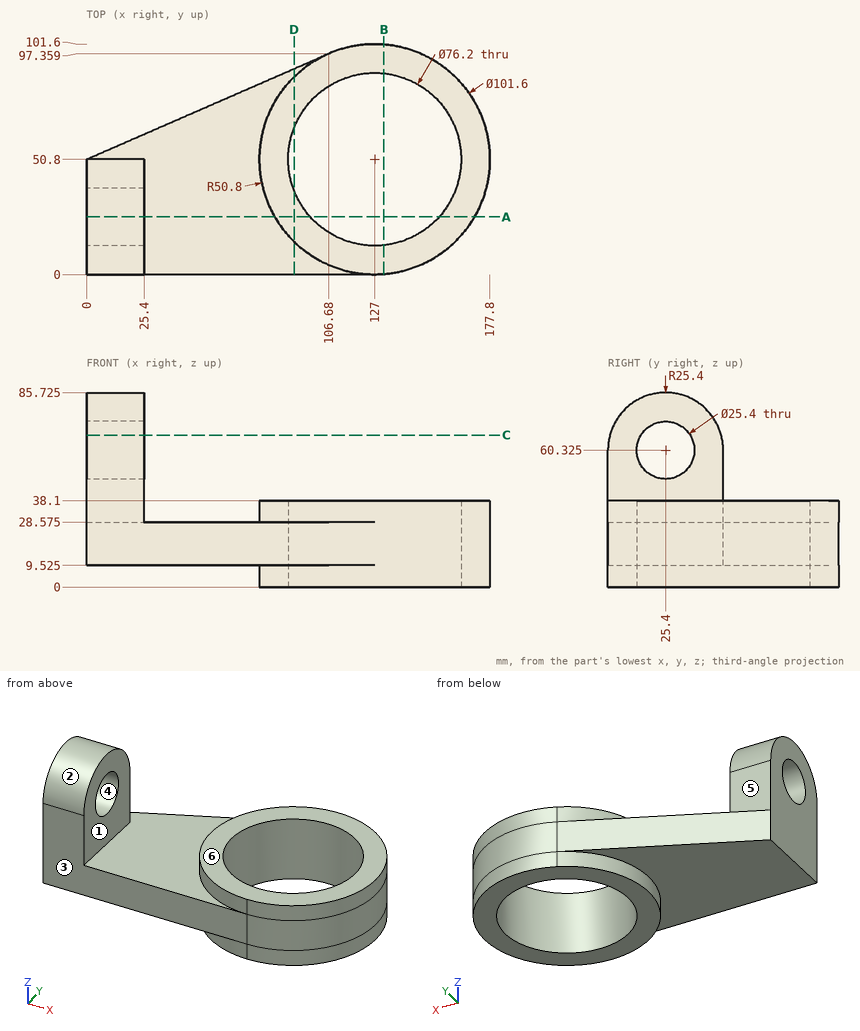
Design review of the part shown in the three views and the two pictorial views. Dimensions are in mm from the part's minimum x, y and z. A direction names the side the tool comes from. Coordinates: 2 decimals unless noted, no trailing zeros. Order: outer loops, then holes, each group sorted by start corner. A loop starts at its lowest first (then second) coordinate and runs counter-clockwise, first axis right, second up. Notation, with made-up numbers: (-2.5, 85.5) -> (39.5, 85.5) arc R21 ccw to (39.5, 106.5) -> close; hole circle Ø7 at (41, 42). An arc over 180 degrees is marked (long way). Use one line per item in the form item = value. Start each with the question number.
(1) The part is to be moulded in two halves that separate along Y. For the marked faces 3, 4, 5 and 6, say which applies: +Y half, -Y half, draft (parallel to the pull), parting line (faces both ways), or undercut.
(2) Insertion check: pin 1 (6 mm diameter, centred on x = 56, y = 54, fed in from -Z) (3 decimals); pin 2 (6 mm diameter, centred on y = 31, z = 10, fed in from +X); pin 3 (4 mm diameter, centred on x = 67, y = 54.5, fed in from +Z) (3 decimals); pin 4 (8 mm diameter, centred on x = 57, y = 82, fed in from -Z). Each pin has a flat end and moves straight along its axis. Give the tip position at first contact, or say it passes through.
(3) Add section A-A on y = 25.4. State the section outline as (x, z) points (3 decimals), plus the area to 3 significant figures.
(4) For probe 1 along X at (y, z) = (50.8, 11); probe 2 along Z at (x, y) = (11, 25) (3 decimals); probe 3 along Z at (x, y) = (159.5, 16.5), list the stretches that pass through material, from the lowest coordinate up.
(5) Add section D-D on x = 91.5. State the section outline as (y, z) points (3 decimals).
(6) Add section B-B on x = 131. State the section outline as (y, z) points (1 decimal), plus the area to 3 significant figures.
(7) Add section C-C on z = 67. State the section outline as (x, y) points.
(8) For the marked faces 1 and 2, list the 3-axis set-ups (+Z, -Z, +X, -X, +Y, -Y) from which the entire face can be reached by the end or side of a thin tool; tool diameter is ignored.
Answer block:
q1.face_3 = -Y half
q1.face_4 = undercut
q1.face_5 = +Y half
q1.face_6 = draft
q2.pin_1 = 9.525
q2.pin_2 = 174.94
q2.pin_3 = 28.575
q2.pin_4 = through
q3.outline = (0, 9.525) -> (83.006, 9.525) -> (83.006, 0) -> (98.602, 0) -> (98.602, 38.1) -> (83.006, 38.1) -> (83.006, 28.575) -> (25.4, 28.575) -> (25.4, 47.625) -> (0, 47.625) -> close; (0, 73.025) -> (25.4, 73.025) -> (25.4, 85.725) -> (0, 85.725) -> close; (155.398, 0) -> (170.994, 0) -> (170.994, 28.575) -> (170.994, 38.1) -> (155.398, 38.1) -> close
q3.area = 3,580 mm²
q4.probe_1 = 0 to 88.9, 165.1 to 177.8
q4.probe_2 = 9.525 to 47.631, 73.019 to 85.722
q4.probe_3 = 0 to 38.1
q5.outline = (0, 9.525) -> (14.463, 9.525) -> (14.463, 0) -> (36.967, 0) -> (36.967, 38.1) -> (14.463, 38.1) -> (14.463, 28.575) -> (0, 28.575) -> close; (64.633, 0) -> (87.137, 0) -> (87.137, 9.525) -> (90.734, 9.525) -> (90.734, 28.575) -> (87.137, 28.575) -> (87.137, 38.1) -> (64.633, 38.1) -> close
q6.outline = (0.2, 0) -> (12.9, 0) -> (12.9, 38.1) -> (0.2, 38.1) -> close; (88.7, 0) -> (101.4, 0) -> (101.4, 28.6) -> (101.4, 38.1) -> (88.7, 38.1) -> close
q6.area = 972 mm²
q7.outline = (0, 0.89) -> (25.4, 0.89) -> (25.4, 14.6) -> (0, 14.6) -> close; (0, 36.2) -> (25.4, 36.2) -> (25.4, 49.91) -> (0, 49.91) -> close
q8.face_1 = +Z, +Y, -Y
q8.face_2 = +Z, +X, -X
